Check sheet for the modelled part. Datum: model origin and axes. Units: mm. A direction names the side the tool comes from. Coordinates: 2 decimals unless noted, no trailing zeros.
1. Gauge pin test, flat ends, axial feed: pin 1 Ø5 at (x, z) = (-6.5, 33.5) entering from -Y; pin 2 Ø1.8 at (x, y) = (12, 12) entering from +Z; pin 3 Ø3.5 at (x, y) = (7.5, 9.5) entering from +Z. Record the tip position at first contact, or that the pin passes through.
2. Set-up check for faces 1 (the cylindrical face through (-14.1, 14.14, 1.52)), 2 (the flat face through (-10.3, 12.4, 3)), 3 (the flat face through (-14, -12, 3)), 4 (the cylindrical face through (-11.99, 0.53, 6.41)): record each of +Z, -Z, +X, -X, +Y, -Y from which the full face is reachable in a straight line by a thin tool's end or side.
3. Draft check along Z on faces 5 (the flat face through (0, 15, 1)), 6 (the cylindrical face through (-1.757, 45.07, 39.615)), 7 (the cylindrical face through (-2.601, 45.07, 64.715)). Enter one of: released by +Z, released by -Z, zero draft, split by the parting line, or undercut.
4. Thickness scan on line 1 (Z direction, x = 0, y = 45.25); line 2 (Y direction, x = 0, z = 3.5); line 3 (X direction, y = -7, z = 5). Record the ranges inside material, lowest first.
```python
from build123d import *

# Parameters (mm, degrees)
ESQUISSE1_W        = 30
ESQUISSE1_H        = 30
ESQUISSE1_R        = 12
ESQUISSE1_R_2      = 1.5
BOSS_EXTRU_1_DEPTH = 3
ESQUISSE4_R        = 13.5
ESQUISSE4_R_2      = 12
CONG_1_R           = 2
CONG_2_R           = 3


with BuildPart() as part:
    # Esquisse1 → Boss.-Extru.1 (new body)
    with BuildSketch(Plane.XY):
        Rectangle(ESQUISSE1_W, ESQUISSE1_H)
        Circle(ESQUISSE1_R, mode=Mode.SUBTRACT)
        with Locations((-12, 12)):
            Circle(ESQUISSE1_R_2, mode=Mode.SUBTRACT)
        with Locations((12, 12)):
            Circle(ESQUISSE1_R_2, mode=Mode.SUBTRACT)
        with Locations((12, -12)):
            Circle(ESQUISSE1_R_2, mode=Mode.SUBTRACT)
        with Locations((-12, -12)):
            Circle(ESQUISSE1_R_2, mode=Mode.SUBTRACT)
    extrude(amount=BOSS_EXTRU_1_DEPTH)

    # Balayage-Mince1: sweep along a path in Esquisse2
    with BuildLine(Plane(origin=(0, 0, 0), x_dir=(0, 0, -1), z_dir=(1, 0, 0))) as balayage_mince1_path:
        Line((-3, 0), (-13, 0))
        ThreePointArc((-13, 0), (-41.284271247, 11.715728753), (-53, 40))
        Line((-53, 40), (-53, 50))
    # Esquisse4 → Balayage-Mince1 (sweep)
    with BuildSketch(Plane.XY.offset(3)):
        Circle(ESQUISSE4_R)
        Circle(ESQUISSE4_R_2, mode=Mode.SUBTRACT)
    sweep(path=balayage_mince1_path.line)

    # Congé1
    cong_1_edges = [part.edges().sort_by_distance(p)[0] for p in [
        (-13.5, 0, 3),
    ]]
    fillet(cong_1_edges, radius=CONG_1_R)

    # Congé2
    cong_2_edges = [part.edges().sort_by_distance(p)[0] for p in [
        (15, -15, 1.5),
        (-15, -15, 1.5),
        (-15, 15, 1.5),
        (15, 15, 1.5),
    ]]
    fillet(cong_2_edges, radius=CONG_2_R)


solid = part.part
```
Data:
1. pin 1: stops at y = -9.2
1. pin 2: stops at z = 51.72
1. pin 3: stops at z = 55.94
2. face 1: -Z, -X, +Y
2. face 2: -X, +Y
2. face 3: +Z, -X, -Y
2. face 4: -Z
3. face 5: zero draft
3. face 6: split by the parting line
3. face 7: undercut
4. line 1: z = 39.5 to 41, 65 to 66.5
4. line 2: y = -14.11 to -12, 12 to 14.11
4. line 3: x = -11.54 to -9.75, 9.75 to 11.54
